Check sheet for the modelled part. Datum: model origin and axes. Units: mm. A direction names the side the tool comes from. Give positions to 0.01 mm unless a question says otherwise; leave off trailing zeros. Write each loop counter-clockwise with the first axis right and the second up, starting at its lowest first coordinate (ties: lowest second). Pieces come first, ordered by that corner, then holes. Notation, with made-up numbers: (57, 18.5) -> (95, 18.5) arc R30 ccw to (95, 40.5) -> close; hole circle Ø8 at (43.5, 50). An arc over 180 degrees is marked (long way). Use a Markdown table: item, result. Add a question column.
1. Gauge pin test, flat ends, axial feed: P1, Ø3, axis at y = -61.5, z = 5, coming from the -X side; P2, Ø10, axis at x = 15.5, y = 36.5, coming from the -Z side; P3, Ø4, axis at y = -66.5, z = -32, coming from the +X side; P4, Ø10, axis at y = -148, z = -16, coming from the -X side. Record the tip position at first contact, or that the pin passes through.
2. Scan lines: probe 1 along Y at (x, z) = (14, 25.5) (3 decimals); probe 2 along X at (y, z) = (-102, 18); probe 3 along X at (y, z) = (-34, 2). Record each from-to range of solid material in increasing order. Write a range as [from, to].
3. Set-up check for faces 1 (the flat face through (0, -200.025, 0)), 2 (the cylindrical face through (42.397, -58.093, -13.352)): record each of +Z, -Z, +X, -X, +Y, -Y from which the full face is reachable in a straight line by a thin tool's end or side.
4. Cross-section at A-A (y = 4). Enter the section's corners in (x, z), then the cut area to 3 significant figures.
Autodesk Inventor part; units mm, degrees
ref_plane "YZ Plane" through (0, 0, 0) normal (1, 0, 0) x (0, 1, 0)
ref_plane "XZ Plane" through (0, 0, 0) normal (0, 1, 0) x (-1, 0, 0)
ref_plane "XY Plane" through (0, 0, 0) normal (0, 0, 1) x (1, 0, 0)
sketch "Sketch1" plane through (0, 0, 0) normal (0, 1, 0) x (-1, 0, 0)
  circle A0 centre (0, 0) radius 50.8
  dimension "d0" = 101.6
extrude "Extrusion1" add sketch "Sketch1" along normal blind 88.9
fillet "Fillet1" radius 10.16 1 edges at (50.8, 88.9, 0)
sketch "Sketch2" plane through (0, 0, 0) normal (0, -1, 0) x (1, 0, 0)
  circle A0 centre (0, 0) radius 50.8
  circle A1 centre (0, 0) radius 44.45
  dimension "d4" = 88.9
extrude "Extrusion2" add sketch "Sketch2" along normal blind 12.7 contours A1
loft "Loft1" add section 1 edges at (50.8, 0, 0) section 2 edges at (-44.45, -12.7, 0)
fillet "Fillet2" radius 5.08 1 edges at (50.8, 0, 0)
sketch "Sketch3" plane through (0, -12.7, 0) normal (0, -1, 0) x (1, 0, 0)
  circle A0 centre (0, 0) radius 44.45
extrude "Extrusion3" add sketch "Sketch3" along normal blind 92.075
sketch "Sketch4" plane through (0, -104.775, 0) normal (0, -1, 0) x (1, 0, 0)
  circle A0 centre (0, 0) radius 44.45
  circle A1 centre (0, 0) radius 9.525
  dimension "d14" = 19.05
extrude "Extrusion4" add sketch "Sketch4" along normal blind 38.1 contours A1
sketch "Sketch5" plane through (0, -142.875, 0) normal (0, -1, 0) x (1, 0, 0)
  circle A0 centre (0, 0) radius 9.525
  circle A1 centre (0, 0) radius 3.175
  dimension "d17" = 6.35
extrude "Extrusion5" add sketch "Sketch5" along normal blind 57.15 contours A1
properties part number "1617evs"
Worked answers:
| question | item | result |
|---|---|---|
| 1 | P1 | stops at x = -44.31 |
| 1 | P2 | stops at z = -49.7 |
| 1 | P3 | stops at x = 32.8 |
| 1 | P4 | passes through |
| 2 | probe 1 | y = [-104.775, 88.9] |
| 2 | probe 2 | x = [-40.64, 40.64] |
| 2 | probe 3 | x = [-44.4, 44.4] |
| 3 | face 1 | +Z, -Z, +X, -X, -Y |
| 3 | face 2 | -Y |
| 4 | outline | circle Ø101.6 at (0, 0) |
| 4 | area | 8,110 mm² |
